The listing builds one solid part. Answer for the finished solid, in the listing's coordinates (mm). A direction names the side the tool comes from. Give positions to 0.01 mm unless a question says otherwise; leave off trailing zeros. Loops run counter-clockwise (first coordinate to the right, second up) from the corner with the lowest first, then second, coordinate; pieces in that order, holes last. Notation, with made-up numbers: M 71,-6 L 102,-6 A25 ccw 102,27 Z; hole C -9.5,54 d5. An arc over 180 degrees is marked long. Return JSON: item names as keys, results as strings.
from build123d import *

# Parameters (mm, degrees)
F1_DEPTH = 36.2
F2_W     = 61.498966068
F2_H     = 68.6773248017
F3_DEPTH = 24


with BuildPart() as f1:
    # F0 (on Top) → F1 (new body, symmetric)
    with BuildSketch(Plane.XY):
        Polygon((50.3633767366, 24.2659896612), (50.3633767366, 44.4113351405), (-50.3633767366, 44.4113351405), (-50.3633767366, -44.4113351405), (-29.0734022856, -44.4113351405), (-29.0734022856, 24.2659896612), align=None)
    extrude(amount=F1_DEPTH, both=True)

    # F2 (on face) → F3 (join)
    with BuildSketch(Plane(origin=(0, 0, -36.2), x_dir=(1, 0, 0), z_dir=(0, 0, -1))):
        with Locations((1.6760807484, 10.0726727396)):
            Rectangle(F2_W, F2_H)
    extrude(amount=-F3_DEPTH)


solid = f1.part
(1) Determine the mould class of faces 1 (the flat face through (-19, -44.411, -17)), 2 (the flat face through (-12, -1, -36.2)), 3 (the flat face through (1, -11, -12.2)) for opening direction Z: released by +Z, released by -Z, zero draft, split by the parting line, or undercut.
Values follow:
{"face 1": "zero draft", "face 2": "released by -Z", "face 3": "released by +Z"}
(2) A tool of negligible diameter and unlimited length cuts with its end or side. For faces 4 (the flat face through (-29.073, -11, 12)), 5 (the flat face through (32.426, -10, -24)), 6 (the flat face through (-23, 30, 36.2)), from which of +Z, -Z, +X, -X, +Y, -Y can it reach the whole face along a straight path? Write none if from no direction.
Values follow:
{"face 4": "+Z, +X, -Y", "face 5": "+Z, -Z, +X, -Y", "face 6": "+Z, +X, -X, +Y, -Y"}
(3) The part is cut by section B-B (y = -2.5). Determine the outline of the cut face in (x, z), and give its area (3 significant figures).
Values follow:
{"outline": "M -50.36,-36.2 L 32.43,-36.2 L 32.43,-12.2 L -29.07,-12.2 L -29.07,36.2 L -50.36,36.2 Z", "area": "3,020 mm²"}
(4) The part is cut by section A-A (z = 16). Determine the outline of the cut face in (x, y), and give its area (3 significant figures).
Values follow:
{"outline": "M -50.36,-44.41 L -29.07,-44.41 L -29.07,24.27 L 50.36,24.27 L 50.36,44.41 L -50.36,44.41 Z", "area": "3,490 mm²"}
(5) Straight lines are drawn through the part: line 1 along X through (y, z) = (-16.5, 27); line 2 along Y through (x, z) = (2, 14.5); line 3 along Z through (x, y) = (1.5, -27). For each, find the intervals that lie inside material, in ascending order.
Values follow:
{"line 1": "-50.36 to -29.07", "line 2": "24.27 to 44.41", "line 3": "-36.2 to -12.2"}
(6) Given pin 1 (2 mm diameter, centred on x = 2, z = 21, fed in from -Y); pin 2 (10 mm diameter, centred on y = -5.5, z = -3, fed in from +X), each flat-ended and moving along its own axis, determine where each tip first touches the part or whether it passes through.
Values follow:
{"pin 1": "y = 24.27", "pin 2": "x = -29.07"}
